Source: CAD feature listing. Evaluate the final solid. Frame: model axes, mm. A direction names the side the tool comes from. Round coordinates to 2 decimals unless told otherwise and drop trailing zeros. Order: outer loops, then holes, each group sorted by start corner. A loop starts at its lowest first (then second) coordinate and runs counter-clockwise, first axis right, second up. Notation, with made-up numbers: (41.5, 71) - (64.5, 71) arc R11 cw to (64.5, 82) - close; hole circle Ø3 at (59.5, 49.25). An arc over 180 degrees is marked (long way). Return JSON: item names as keys, results as strings. Group by question number.
1) Section B-B, the plane y = 24.5. Return loops of the section in (x, z).
2) Access query for faces 1 (the flat face through (28.663, 11.18, -12.522)), 2 (the flat face through (28, 11, -25.4)). Directions: +Z, -Z, +X, -X, +Y, -Y. A direction counts if a zero-diameter tool reaches every point of the face in a straight line with its end or side. Return the directions, or none.
3) Section C-C, the plane x = 11.5. Return loops of the section in (y, z).
4) Section A-A, the plane x = 15.5. Return loops of the section in (y, z).
5) Ray query, line 1 (Y direction, x = 20.5, z = -8.25); line 2 (Y direction, x = 24.25, z = -4.25); line 3 (X direction, y = 23.5, z = -5.25). Return the intervals inside material, ascending. Write a range as from..to.
6) Section D-D, the plane x = 33. Return loops of the section in (y, z).
7) Contact query for flat-ended pins moving along their axis: P1, Ø4, axis at x = 13, z = -10, coming from the -Y side; P2, Ø8, axis at y = 26, z = -17, coming from the -X side; P3, Ø8, axis at x = 14, z = -16, coming from the -Y side; P4, Ø3, axis at x = 25.22, y = 9.24, coming from the +Z side. Output: stop coordinate, or through.
8) Mould query, pull axis Y, two halves, no side actions, for faces 3 (the flat face through (18.07, 9.31, -12.52)), 4 (the flat face through (28, 11, 0)), 5 (the cylindrical face through (34.794, 20.357, -12.522)). Classes: pulls with the +Y half, pulls with the -Y half, needs draft (parallel to the pull), parting line crosses it, or undercut.
```python
from build123d import *

# Parameters (mm, degrees)
F0_R     = 13.1466034644
F1_DEPTH = 25.4
F3_DEPTH = 25.4


with BuildPart() as f1:
    # F0 (on Top) → F1 (new body)
    with BuildSketch(Plane.XY):
        with Locations((22.2542323142, 16.408336586)):
            Circle(F0_R)
        with BuildLine():
            ThreePointArc((17.3713553391, 8.1242080796), (17.4837466767, 24.7576922166), (31.8703267742, 16.408336586))
            ThreePointArc((31.8703267742, 16.408336586), (31.2310278998, 12.9606687251), (29.3981352357, 9.9714177802))
            ThreePointArc((29.3981352357, 9.9714177802), (26.7985489054, 7.9337593468), (23.662805616, 6.895966013))
            ThreePointArc((23.662805616, 6.895966013), (20.4117228442, 6.9704114159), (17.3713553391, 8.1242080796))
        make_face(mode=Mode.SUBTRACT)
        with BuildLine():
            ThreePointArc((23.662805616, 6.895966013), (26.7985489054, 7.9337593468), (29.3981352357, 9.9714177802))
            Line((29.3981352357, 9.9714177802), (27.9079406361, 12.4224082931))
            add(Edge.make_bspline(
                [(23.662805616, 10.0813770912), (25.3011567226, 10.4707698937), (26.9352469675, 11.7126964633), (27.9079406361, 12.4224082931)],
                knots=[0.5019879856, 0.5019879856, 0.5019879856, 0.5019879856, 1, 1, 1, 1], degree=3))
            Line((23.662805616, 10.0813770912), (23.662805616, 6.895966013))
        make_face()
        with BuildLine():
            Line((18.7523793429, 10.4672079906), (17.3713553391, 8.1242080796))
            ThreePointArc((17.3713553391, 8.1242080796), (20.4117228442, 6.9704114159), (23.662805616, 6.895966013))
            Line((23.662805616, 6.895966013), (23.662805616, 10.0813770912))
            add(Edge.make_bspline(
                [(18.7523793429, 10.4672079906), (20.3556140754, 10.1625747365), (22.0113744297, 9.688875499), (23.662805616, 10.0813770912)],
                knots=[0, 0, 0, 0, 0.5019879856, 0.5019879856, 0.5019879856, 0.5019879856], degree=3))
        make_face()
    extrude(amount=-F1_DEPTH)

    # F2 (on face) → F3 (cut)
    with BuildSketch(Plane.XY):
        with BuildLine():
            add(Edge.make_bspline(
                [(22.9678027966, 9.964484064), (22.2495247463, 9.8906014768), (21.5319362459, 9.9530967079), (20.8197145148, 10.0668024382)],
                knots=[1.070410353, 1.070410353, 1.070410353, 1.070410353, 1.2887337185, 1.2887337185, 1.2887337185, 1.2887337185], degree=3))
            ThreePointArc((22.9678027966, 9.964484064), (21.9116925702, 10.3921507142), (20.8197145148, 10.0668024382))
        make_face()
        with BuildLine():
            ThreePointArc((20.8197145148, 10.0668024382), (21.046706191, 7.1381420291), (23.551896206, 8.6719607934))
            ThreePointArc((23.551896206, 8.6719607934), (23.3990939232, 9.3811472139), (22.9678027966, 9.964484064))
            add(Edge.make_bspline(
                [(22.9678027966, 9.964484064), (22.2495247463, 9.8906014768), (21.5319362459, 9.9530967079), (20.8197145148, 10.0668024382)],
                knots=[1.070410353, 1.070410353, 1.070410353, 1.070410353, 1.2887337185, 1.2887337185, 1.2887337185, 1.2887337185], degree=3))
        make_face()
        with BuildLine():
            ThreePointArc((25.6390406998, 10.8996020133), (24.5525965747, 10.8191970092), (23.735100283, 10.0991097821))
            add(Edge.make_bspline(
                [(25.6390406998, 10.8996020133), (25.0340333492, 10.5593442342), (24.3856651722, 10.2635991457), (23.735100283, 10.0991097821)],
                knots=[0.7948888634, 0.7948888634, 0.7948888634, 0.7948888634, 0.9926743355, 0.9926743355, 0.9926743355, 0.9926743355], degree=3))
        make_face()
        with BuildLine():
            add(Edge.make_bspline(
                [(25.6390406998, 10.8996020133), (25.0340333492, 10.5593442342), (24.3856651722, 10.2635991457), (23.735100283, 10.0991097821)],
                knots=[0.7948888634, 0.7948888634, 0.7948888634, 0.7948888634, 0.9926743355, 0.9926743355, 0.9926743355, 0.9926743355], degree=3))
            ThreePointArc((23.735100283, 10.0991097821), (24.7720390374, 7.5907286664), (26.9257952006, 9.2425616458))
            ThreePointArc((26.9257952006, 9.2425616458), (26.566331746, 10.2915516272), (25.6390406998, 10.8996020133))
        make_face()
    extrude(amount=-F3_DEPTH, mode=Mode.SUBTRACT)


solid = f1.part
```
Geometry check:
{
 "1": {"outline": "(11.89, -25.4) - (17.06, -25.4) - (17.06, 0) - (11.89, 0) - close; (27.45, -25.4) - (32.62, -25.4) - (32.62, 0) - (27.45, 0) - close"},
 "2": {"face 1": "+Z, -Z", "face 2": "-Z, +X, -X, +Y, -Y"},
 "3": {"outline": "(8.85, -25.4) - (23.97, -25.4) - (23.97, 0) - (8.85, 0) - close"},
 "4": {"outline": "(5.13, -25.4) - (9.56, -25.4) - (9.56, 0) - (5.13, 0) - close; (23.25, -25.4) - (27.69, -25.4) - (27.69, 0) - (23.25, 0) - close"},
 "5": {"line 1": "3.38..7.58, 9.77..10.12, 25.86..29.44", "line 2": "3.41..7.83, 25.82..29.4", "line 3": "11.18..15.76, 28.75..33.32"},
 "6": {"outline": "(8.83, -25.4) - (23.98, -25.4) - (23.98, 0) - (8.83, 0) - close"},
 "7": {"P1": "y = 5.44", "P2": "x = 10.36", "P3": "y = 3.97", "P4": "through"},
 "8": {"face 3": "undercut", "face 4": "needs draft", "face 5": "parting line crosses it"}
}
